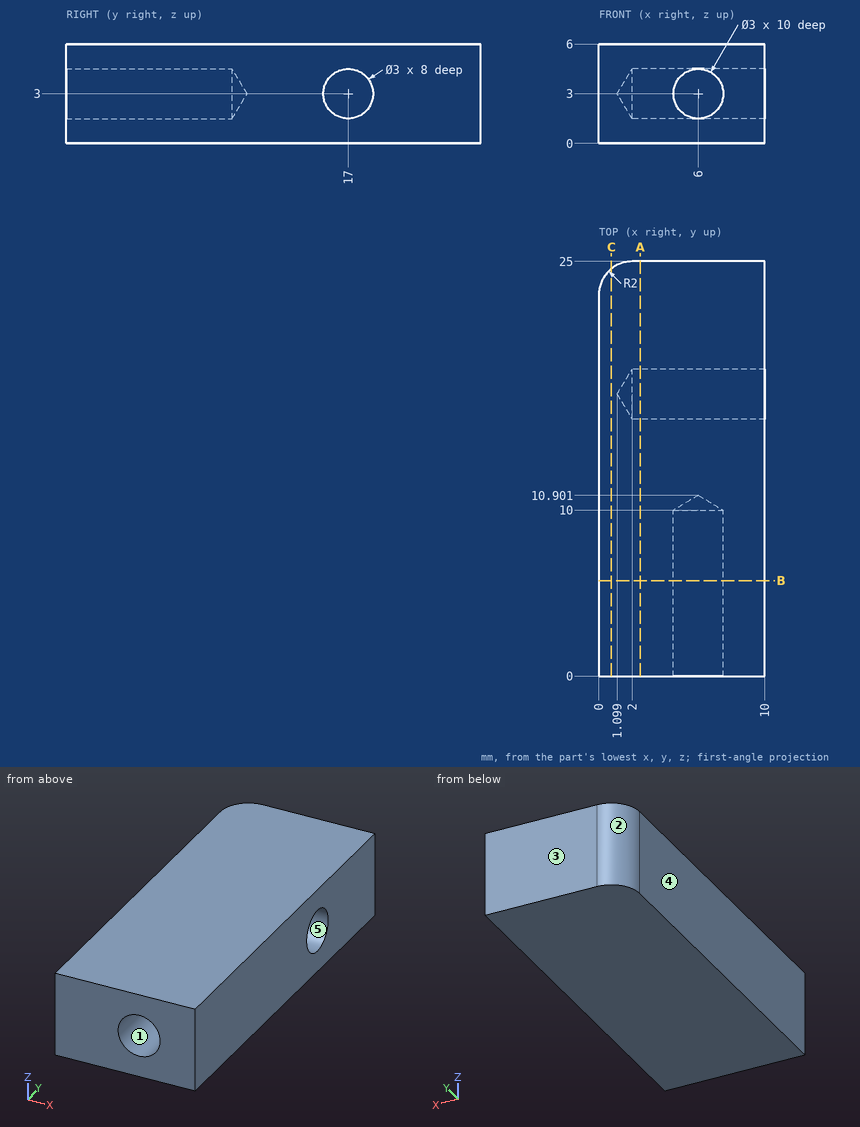
The drawing under review shows one solid part. Ordinate dimensions are in mm from its lowest x, y, z. A direction names the side the tool comes from. Give positions to 0.01 mm unless a question says otherwise; leave off trailing zeros. Order: outer loops, then holes, each group sorted by start corner. A loop starts at its lowest first (then second) coordinate and runs counter-clockwise, first axis right, second up. Notation, with made-up numbers: M 35,1.25 L 90,1.25 A29 ccw 90,25.25 Z; hole C -4.75,7 d11. An arc over 180 degrees is marked long. Answer in a Markdown table with one row per item. Add a question column.
1. Machinability: for the marked faces 1 and 2, which of the approach directions +Z, -Z, +X, -X, +Y, -Y give a long, thin tool a straight path to every point of the face, cutting with its end or side? Answer none if there is none.
2. Add section A-A on x = 2.5. State the section outline as (y, z) points, plus the area to 3 significant figures.
3. To check wall thickness, follow line 1 along Z through (x, y) = (4.75, 17); line 2 along Y through (x, z) = (8.75, 2.95). State the ranges of each line that lie inside material, in increasing order.
4. Mouldability with a two-part tool opening along Y and no side actions: class the marked faces 3, 4 and 5 as released by +Y, released by -Y, zero draft, split by the parting line, or undercut.
5. Add section B-B on y = 5.75. State the section outline as (x, z) points.
6. Add section C-C on x = 0.75. State the section outline as (y, z) points, plus the area to 3 significant figures.
The answers:
| question | item | result |
|---|---|---|
| 1 | face 1 | -Y |
| 1 | face 2 | +Z, -Z, -X, +Y |
| 2 | outline | M 0,0 L 25,0 L 25,6 L 0,6 Z; hole C 17,3 d3 |
| 2 | area | 143 mm2 |
| 3 | line 1 | 0 to 1.5, 4.5 to 6 |
| 3 | line 2 | 0 to 15.5, 18.5 to 25 |
| 4 | face 3 | released by +Y |
| 4 | face 4 | zero draft |
| 4 | face 5 | undercut |
| 5 | outline | M 0,0 L 10,0 L 10,6 L 0,6 Z; hole C 6,3 d3 |
| 6 | outline | M 0,0 L 24.56,0 L 24.56,6 L 0,6 Z |
| 6 | area | 147 mm2 |
